Check sheet for the modelled part. Datum: model origin and axes. Units: mm. A direction names the side the tool comes from. Give positions to 0.01 mm unless a question says otherwise; leave off trailing zeros. Order: outer loops, then holes, each group sorted by start corner. A loop starts at its lowest first (then second) coordinate and runs counter-clockwise, first axis right, second up. Notation, with made-up numbers: (82, 20.25) - (139, 20.25) arc R19 cw to (139, 33.25) - close; hole circle Ø8 at (-17, 38.5). An arc over 180 degrees is marked (long way). Answer in a Markdown table with one row per item.
from build123d import *

# Parameters (mm, degrees)
BOSS_EXTRUDE1_DEPTH      = 3.175
SKETCH2_W                = 78.74
SKETCH2_H                = 6.604
CUT_EXTRUDE1_DEPTH       = 4.175
SKETCH8_W                = 13.97
SKETCH8_H                = 5.08
CUT_EXTRUDE2_DEPTH       = 4.175
FILLET1_R                = 1.27
F_8_CLEARANCE_HOLE1_D    = 4.4958
CIRPATTERN1_COUNT        = 3
FILLET1_OF_CIRPATTERN1_R = 1.27
F_8_CLEARANCE_HOLE2_D    = 4.4958
CIRPATTERN2_COUNT        = 3
F_8_CLEARANCE_HOLE3_D    = 4.4958


with BuildPart() as part:
    # Sketch1 → Boss-Extrude1 (new body)
    with BuildSketch(Plane(origin=(0, 0, 0), x_dir=(1, 0, 0), z_dir=(0, 1, 0))):
        Polygon((48.611580185, -36.986616861), (56.337139895, -23.605554928), (7.725559709, 60.592171789), (-7.725559709, 60.592171789), (-56.337139895, -23.605554928), (-48.611580185, -36.986616861), align=None)
    extrude(amount=-BOSS_EXTRUDE1_DEPTH)

    # Sketch2 → Cut-Extrude1 (cut, through all)
    with BuildSketch(Plane(origin=(0, 0, 0), x_dir=(1, 0, 0), z_dir=(0, 1, 0))):
        with Locations((0, -33.684616861)):
            Rectangle(SKETCH2_W, SKETCH2_H)
    cut_extrude1 = extrude(amount=-CUT_EXTRUDE1_DEPTH, mode=Mode.SUBTRACT)

    # Sketch8 → Cut-Extrude2 (cut, through all)
    with BuildSketch(Plane(origin=(0, 0, 0), x_dir=(1, 0, 0), z_dir=(0, 1, 0))):
        with Locations((-15.24, -27.842616861)):
            Rectangle(SKETCH8_W, SKETCH8_H)
    cut_extrude2 = extrude(amount=-CUT_EXTRUDE2_DEPTH, mode=Mode.SUBTRACT)

    # Fillet1
    fillet1_edges = [part.edges().sort_by_distance(p)[0] for p in [
        (-39.37, -1.5875, 30.382616861),
        (39.37, -1.5875, 30.382616861),
        (-22.225, -1.5875, 30.382616861),
        (-22.225, -1.5875, 25.302616861),
        (-8.255, -1.5875, 25.302616861),
        (-8.255, -1.5875, 30.382616861),
    ]]
    fillet(fillet1_edges, radius=FILLET1_R)

    # 8 Clearance Hole1 (through all)
    with Locations(Plane(origin=(0, 0, 0), x_dir=(1, 0, 0), z_dir=(0, 1, 0))):
        with Locations((-47.780246463, -27.585938157)):
            f_8_clearance_hole1 = Hole(F_8_CLEARANCE_HOLE1_D / 2)

    # CirPattern1: Cut-Extrude1, Cut-Extrude2, 8 Clearance Hole1 ×3 about axis
    cirpattern1_axis = Axis((0, 0, 0), (0, 1, 0))
    for i in range(1, CIRPATTERN1_COUNT):
        add(cut_extrude1.rotate(cirpattern1_axis, i * 360 / CIRPATTERN1_COUNT), mode=Mode.SUBTRACT)
        add(cut_extrude2.rotate(cirpattern1_axis, i * 360 / CIRPATTERN1_COUNT), mode=Mode.SUBTRACT)
        add(f_8_clearance_hole1.rotate(cirpattern1_axis, i * 360 / CIRPATTERN1_COUNT), mode=Mode.SUBTRACT)

    # Fillet1 of CirPattern1
    fillet1_of_cirpattern1_edges = [part.edges().sort_by_distance(p)[0] for p in [
        (45.997118036, -1.5875, 18.904111716),
        (6.627118036, -1.5875, -49.286728578),
        (37.424618036, -1.5875, 4.056106168),
        (33.025208984, -1.5875, 6.596106168),
        (26.040208984, -1.5875, -5.502268723),
        (30.439618036, -1.5875, -8.042268723),
        (-6.627118036, -1.5875, -49.286728578),
        (-45.997118036, -1.5875, 18.904111716),
        (-15.199618036, -1.5875, -34.43872303),
        (-10.800208984, -1.5875, -31.89872303),
        (-17.785208984, -1.5875, -19.800348139),
        (-22.184618036, -1.5875, -22.340348139),
    ]]
    fillet(fillet1_of_cirpattern1_edges, radius=FILLET1_OF_CIRPATTERN1_R)

    # 8 Clearance Hole2 (through all)
    with Locations(Plane(origin=(0, 0, 0), x_dir=(1, 0, 0), z_dir=(0, 1, 0))):
        with Locations((-27.94, -21.59)):
            f_8_clearance_hole2 = Hole(F_8_CLEARANCE_HOLE2_D / 2)

    # CirPattern2: 8 Clearance Hole2 ×3 about axis
    cirpattern2_axis = Axis((0, 0, 0), (0, 1, 0))
    for i in range(1, CIRPATTERN2_COUNT):
        add(f_8_clearance_hole2.rotate(cirpattern2_axis, i * 360 / CIRPATTERN2_COUNT), mode=Mode.SUBTRACT)

    # 8 Clearance Hole3 (through all)
    with Locations(Plane(origin=(0, 0, 0), x_dir=(1, 0, 0), z_dir=(0, 1, 0))):
        with Locations((-6.934384891, 6.286512516), (-3.048, -21.365616861)):
            Hole(F_8_CLEARANCE_HOLE3_D / 2)


solid = part.part
(1) Gauge pin test, flat ends, axial feed: P1, Ø1.6, axis at y = -1.5, z = 33.5, coming from the -X side; P2, Ø1, axis at x = -29.5, y = -1.5, coming from the +Z side; P3, Ø1.5, axis at y = -3, z = 21, coming from the -X side. Record the tip position at first contact, or that the pin passes through.
Geometry says:
| item | result |
|---|---|
| P1 | x = -51.09 |
| P2 | z = 30.38 |
| P3 | x = -55.27 |
(2) Mould release check, pull along Z, two halves, no side actions. Record for faces 1 (the flat face through (-39.37, -2, 34)), 2 (the flat face through (15, -2, 30.383)), 3 (the flat face through (-53.994, -1.565, 19.548)), 4 (the flat face through (10.069, -1.565, -51.274)): pulls with the +Z half, pulls with the -Z half, needs draft (parallel to the pull), parting line crosses it, or undercut.
Geometry says:
| item | result |
|---|---|
| face 1 | needs draft |
| face 2 | pulls with the +Z half |
| face 3 | pulls with the -Z half |
| face 4 | undercut |
(3) Cross-section at D-D, the plane z = -18.5. Record the cut outline in (x, y) (3 decimals).
Geometry says:
| item | result |
|---|---|
| outline | (-24.402, -3.175) - (24.402, -3.175) - (24.402, 0) - (-24.402, 0) - close |
(4) Cross-section at B-B, the plane y = -1.95. Give the number of separate pieces and of enclosed holes in the cut face, then the cut area to 3 significant figures.
Geometry says:
| item | result |
|---|---|
| separate pieces | 1 |
| enclosed holes | 8 |
| area | 4,900 mm² |
(5) Cross-section at A-A, the plane x = -27.94. Record the cut outline in (y, z) (3 decimals).
Geometry says:
| item | result |
|---|---|
| outline | (-3.175, -12.372) - (0, -12.372) - (0, 19.342) - (-3.175, 19.342) - close; (-3.175, 23.838) - (0, 23.838) - (0, 30.383) - (-3.175, 30.383) - close |
(6) Cross-section at C-C, the plane z = -28.5. Record the cut outline in (x, y) (3 decimals).
Geometry says:
| item | result |
|---|---|
| outline | (-12.762, -3.175) - (18.628, -3.175) - (18.628, 0) - (-12.762, 0) - close |
(7) Access from +Z, -Z, +X, -X, +Y, -Y to the whole of each face (thin tool, end or side, straight path). Record for faces 5 (the flat face through (-49.439, -1.565, 16.917)), 6 (the flat face through (-10.862, -1.565, -41.951)), 7 (the flat face through (0, -2, -60.592)), 8 (the cylindrical face through (31.459, -1.61, 11.506)), 9 (the flat face through (-22.225, -2, 28)).
Geometry says:
| item | result |
|---|---|
| face 5 | -Z, +Y, -Y |
| face 6 | -X, +Y, -Y |
| face 7 | -Z, +X, -X, +Y, -Y |
| face 8 | +Y, -Y |
| face 9 | +Z, +Y, -Y |
(8) Thickness scan on L1, parallel to Z at x = -27.94, y = -1.9; L2, parallel to Z at x = -7.5, y = -2.35; L3, parallel to X at y = -0.05, z = 21. Record the ranges inside material, lowest first.
Geometry says:
| item | result |
|---|---|
| L1 | -12.37 to 19.34, 23.84 to 30.38 |
| L2 | -60.59 to -49.75, -47.77 to -8.46, -4.11 to 30.27 |
| L3 | -54.83 to -30.11, -25.77 to -5.27, -0.83 to 54.83 |
